```python
from build123d import *

# Parameters (mm, degrees)
SKETCH3_R            = 31
SKETCH3_R_2          = 1.6
SERVO_MOUNT_DEPTH    = 2
SKETCH4_R            = 31
SKETCH4_R_2          = 24
SPACER_DEPTH         = 9.3
FLEX_CABLE_REACH     = 47.274
SKETCH5_W            = 17
SKETCH5_H            = 0.8
SKETCH7_W            = 24
SKETCH7_H            = 62
CUT_EXTRUDE3_DEPTH   = 45.816180114
SKETCH8_W            = 62
SKETCH8_H            = 24
CUT_EXTRUDE4_DEPTH   = 45.816180114
MOUNTING_HOLES_REACH = 47.274
SKETCH10_R           = 1.4
CUT_EXTRUDE5_REACH   = 46.816
FILLET2_R            = 5


with BuildPart() as part:
    # Sketch3 → Servo mount (new body)
    with BuildSketch(Plane(origin=(0, 0, 0), x_dir=(1, 0, 0), z_dir=(0, 1, 0))):
        with Locations(Location((0, 0, 0), (0, 0, 270))):
            Circle(SKETCH3_R)
        with Locations(Location((0, -8.65, 0), (0, 0, 270))):
            Circle(SKETCH3_R_2, mode=Mode.SUBTRACT)
        with Locations(Location((0, 19.05, 0), (0, 0, 270))):
            Circle(SKETCH3_R_2, mode=Mode.SUBTRACT)
        Polygon((-6.2, 16.1), (-6.2, 2.227105745), (-6.2, -6.4), (-5.7, -6.4), (5.7, -6.4), (6.2, -6.4), (6.2, 2.227105745), (6.2, 16.1), (6.2, 16.8), (5.7, 16.8), (-5.7, 16.8), (-6.2, 16.8), align=None, mode=Mode.SUBTRACT)
    extrude(amount=-SERVO_MOUNT_DEPTH)

    # Sketch4 → Spacer (add)
    with BuildSketch(Plane(origin=(0, -2, 0), x_dir=(-1, 0, 0), z_dir=(0, -1, 0))):
        with Locations(Location((0, 0, 0), (0, 0, 270))):
            Circle(SKETCH4_R)
        with Locations(Location((0, 0, 0), (0, 0, 270))):
            Circle(SKETCH4_R_2, mode=Mode.SUBTRACT)
    extrude(amount=SPACER_DEPTH)

    # Sketch5 → Flex cable (cut, up to next)
    with BuildSketch(Plane(origin=(0, 0, 0), x_dir=(1, 0, 0), z_dir=(0, 1, 0)), mode=Mode.PRIVATE) as flex_cable_sk1:
        with Locations((0, -19.15054858)):
            Rectangle(SKETCH5_W, SKETCH5_H)
    flex_cable_tool1 = extrude(flex_cable_sk1.sketch, amount=-FLEX_CABLE_REACH, mode=Mode.PRIVATE) & part.part
    add(flex_cable_tool1.solids().sort_by_distance((0, 0, 19.150549))[0], mode=Mode.SUBTRACT)

    # Sketch7 → Cut-Extrude3 (cut, through all)
    with BuildSketch(Plane.XZ.offset(2)):
        Rectangle(SKETCH7_W, SKETCH7_H)
    extrude(amount=CUT_EXTRUDE3_DEPTH, mode=Mode.SUBTRACT)

    # Sketch8 → Cut-Extrude4 (cut, through all)
    with BuildSketch(Plane.XZ.offset(2)):
        Rectangle(SKETCH8_W, SKETCH8_H)
    extrude(amount=CUT_EXTRUDE4_DEPTH, mode=Mode.SUBTRACT)

    # Sketch10 → Mounting holes (cut, up to next)
    with BuildSketch(Plane.XZ.offset(11.3), mode=Mode.PRIVATE) as mounting_holes_sk1:
        with Locations(Location((-19.445436483, -19.445436483, 0), (0, 0, 270))):
            Circle(SKETCH10_R)
    mounting_holes_tool1 = extrude(mounting_holes_sk1.sketch, amount=-MOUNTING_HOLES_REACH, mode=Mode.PRIVATE) & part.part
    # Sketch10 → Mounting holes (cut, up to next)
    with BuildSketch(Plane.XZ.offset(11.3), mode=Mode.PRIVATE) as mounting_holes_sk2:
        with Locations(Location((19.445436483, -19.445436483, 0), (0, 0, 270))):
            Circle(SKETCH10_R)
    mounting_holes_tool2 = extrude(mounting_holes_sk2.sketch, amount=-MOUNTING_HOLES_REACH, mode=Mode.PRIVATE) & part.part
    # Sketch10 → Mounting holes (cut, up to next)
    with BuildSketch(Plane.XZ.offset(11.3), mode=Mode.PRIVATE) as mounting_holes_sk3:
        with Locations(Location((-19.445436483, 19.445436483, 0), (0, 0, 270))):
            Circle(SKETCH10_R)
    mounting_holes_tool3 = extrude(mounting_holes_sk3.sketch, amount=-MOUNTING_HOLES_REACH, mode=Mode.PRIVATE) & part.part
    # Sketch10 → Mounting holes (cut, up to next)
    with BuildSketch(Plane.XZ.offset(11.3), mode=Mode.PRIVATE) as mounting_holes_sk4:
        with Locations(Location((19.445436483, 19.445436483, 0), (0, 0, 270))):
            Circle(SKETCH10_R)
    mounting_holes_tool4 = extrude(mounting_holes_sk4.sketch, amount=-MOUNTING_HOLES_REACH, mode=Mode.PRIVATE) & part.part
    add(mounting_holes_tool1.solids().sort_by_distance((-19.445436, -11.3, -19.445436))[0], mode=Mode.SUBTRACT)
    add(mounting_holes_tool2.solids().sort_by_distance((19.445436, -11.3, -19.445436))[0], mode=Mode.SUBTRACT)
    add(mounting_holes_tool3.solids().sort_by_distance((-19.445436, -11.3, 19.445436))[0], mode=Mode.SUBTRACT)
    add(mounting_holes_tool4.solids().sort_by_distance((19.445436, -11.3, 19.445436))[0], mode=Mode.SUBTRACT)

    # Sketch11 → Cut-Extrude5 (cut, up to next)
    with BuildSketch(Plane.XZ.offset(2), mode=Mode.PRIVATE) as cut_extrude5_sk1:
        with BuildLine():
            Line((-12, -22.784609691), (12, -22.784609691))
            Line((12, -22.784609691), (12, -28.583211856))
            ThreePointArc((12, -28.583211856), (0, -31), (-12, -28.583211856))
            Line((-12, -28.583211856), (-12, -22.784609691))
        make_face()
    cut_extrude5_tool1 = extrude(cut_extrude5_sk1.sketch, amount=-CUT_EXTRUDE5_REACH, mode=Mode.PRIVATE) & part.part
    # Sketch11 → Cut-Extrude5 (cut, up to next)
    with BuildSketch(Plane.XZ.offset(2), mode=Mode.PRIVATE) as cut_extrude5_sk2:
        with BuildLine():
            Line((28.583211856, 12), (20.784609691, 12))
            Line((20.784609691, 12), (20.784609691, -12))
            Line((20.784609691, -12), (28.583211856, -12))
            ThreePointArc((28.583211856, -12), (31, 0), (28.583211856, 12))
        make_face()
    cut_extrude5_tool2 = extrude(cut_extrude5_sk2.sketch, amount=-CUT_EXTRUDE5_REACH, mode=Mode.PRIVATE) & part.part
    # Sketch11 → Cut-Extrude5 (cut, up to next)
    with BuildSketch(Plane.XZ.offset(2), mode=Mode.PRIVATE) as cut_extrude5_sk3:
        with BuildLine():
            Line((-28.583211856, -12), (-20.784609691, -12))
            Line((-20.784609691, -12), (-20.784609691, 12))
            Line((-20.784609691, 12), (-28.583211856, 12))
            ThreePointArc((-28.583211856, 12), (-31, 0), (-28.583211856, -12))
        make_face()
    cut_extrude5_tool3 = extrude(cut_extrude5_sk3.sketch, amount=-CUT_EXTRUDE5_REACH, mode=Mode.PRIVATE) & part.part
    # Sketch11 → Cut-Extrude5 (cut, up to next)
    with BuildSketch(Plane.XZ.offset(2), mode=Mode.PRIVATE) as cut_extrude5_sk4:
        with BuildLine():
            Line((12, 20.784609691), (12, 28.583211856))
            ThreePointArc((12, 28.583211856), (0, 31), (-12, 28.583211856))
            Line((-12, 28.583211856), (-12, 20.784609691))
            Line((-12, 20.784609691), (12, 20.784609691))
        make_face()
    cut_extrude5_tool4 = extrude(cut_extrude5_sk4.sketch, amount=-CUT_EXTRUDE5_REACH, mode=Mode.PRIVATE) & part.part
    add(cut_extrude5_tool1.solids().sort_by_distance((0, -2, -26.530561))[0], mode=Mode.SUBTRACT)
    add(cut_extrude5_tool2.solids().sort_by_distance((25.523226, -2, 0))[0], mode=Mode.SUBTRACT)
    add(cut_extrude5_tool3.solids().sort_by_distance((-25.523226, -2, 0))[0], mode=Mode.SUBTRACT)
    add(cut_extrude5_tool4.solids().sort_by_distance((0, -2, 25.523226))[0], mode=Mode.SUBTRACT)

    # Fillet2
    # the kernel refuses this fillet: 5 mm, written as the material it takes off along each edge
    with BuildSketch(Plane(origin=(12, -35.215595033, 28.583211856), x_dir=(0.8512708603213988, -2.9625112876132807e-14, -0.5247265215020731), z_dir=(0, 1, 0))) as fillet2_piece_1:
        with BuildLine():
            CenterArc((8.794767206, 4.940124775), FILLET2_R, 160.140208495, 118.735653745)
            Line((4.092133387, 6.638722774), (0, 0))
            ThreePointArc((0, 0), (4.783119007, -0.371226395), (9.566238013, 0))
        make_face()
    extrude(amount=59.131190067, mode=Mode.SUBTRACT)
    with BuildSketch(Plane(origin=(12, 23.915595033, -28.583211856), x_dir=(0, 0, 1), z_dir=(0, -1, 0))) as fillet2_piece_2_section:
        with BuildLine():
            CenterArc((8.820231871, -4.894514557), FILLET2_R, 101.790043136, 118.735653745)
            ThreePointArc((5.019658797, -8.143459664), (2.193815186, -4.266522167), (0, 0))
            Line((0, 0), (7.798602165, 0))
        make_face()
    fillet2_piece_2 = extrude(amount=59.131190067, mode=Mode.PRIVATE)
    fillet2_piece_2 = split(fillet2_piece_2, bisect_by=Plane(origin=(16.358047436, -1, -22.784609691), z_dir=(0, 0, -1)), keep=Keep.TOP, mode=Mode.PRIVATE)
    add(fillet2_piece_2, mode=Mode.SUBTRACT)
    with BuildSketch(Plane(origin=(12, 23.915595033, -28.583211856), x_dir=(0, 0, 1), z_dir=(0, -1, 0))) as fillet2_piece_3_section:
        with BuildLine():
            CenterArc((8.820231871, -4.894514557), FILLET2_R, 101.790043136, 118.735653745)
            ThreePointArc((5.019658797, -8.143459664), (2.193815186, -4.266522167), (0, 0))
            Line((0, 0), (7.798602165, 0))
        make_face()
    fillet2_piece_3 = extrude(amount=59.131190067, mode=Mode.PRIVATE)
    fillet2_piece_3 = split(fillet2_piece_3, bisect_by=Plane(origin=(12.335072, -2, -21.839415291), z_dir=(0, -1, 0)), keep=Keep.TOP, mode=Mode.PRIVATE)
    add(fillet2_piece_3, mode=Mode.SUBTRACT)
    with BuildSketch(Plane(origin=(28.583211856, 23.915595033, -12), x_dir=(-1, 0, 0), z_dir=(0, -1, 0))) as fillet2_piece_4:
        with BuildLine():
            CenterArc((8.820231871, 4.894514557), FILLET2_R, 139.474303119, 118.735653745)
            ThreePointArc((5.019658797, 8.143459664), (2.193815186, 4.266522167), (0, 0))
            Line((0, 0), (7.798602165, 0))
        make_face()
    extrude(amount=59.131190067, mode=Mode.SUBTRACT)
    with BuildSketch(Plane(origin=(-28.583211856, 23.915595033, -12), x_dir=(1, 0, 0), z_dir=(0, -1, 0)), Plane(origin=(28.583211856, 23.915595033, 12), x_dir=(-1, 0, 0), z_dir=(0, -1, 0))) as fillet2_piece_5:
        with BuildLine():
            CenterArc((8.820231871, -4.894514557), FILLET2_R, 101.790043136, 118.735653745)
            ThreePointArc((5.019658797, -8.143459664), (2.193815186, -4.266522167), (0, 0))
            Line((0, 0), (7.798602165, 0))
        make_face()
    extrude(amount=59.131190067, mode=Mode.SUBTRACT)
    with BuildSketch(Plane(origin=(-28.583211856, 23.915595033, 12), x_dir=(0.5247265215020732, -2.488832337515826e-14, 0.8512708603213986), z_dir=(0, -1, 0)), Plane(origin=(-12, -35.215595033, 28.583211856), x_dir=(-0.8512708603213989, -3.062415803150537e-14, -0.524726521502073), z_dir=(0, 1, 0))) as fillet2_piece_6:
        with BuildLine():
            CenterArc((8.794767206, -4.940124775), FILLET2_R, 81.12413776, 118.735653745)
            Line((4.092133387, -6.638722774), (0, 0))
            ThreePointArc((0, 0), (4.783119007, 0.371226395), (9.566238013, 0))
        make_face()
    extrude(amount=59.131190067, mode=Mode.SUBTRACT)
    with BuildSketch(Plane(origin=(-12, 23.915595033, -28.583211856), x_dir=(-0.8512708603213988, 1.214076701840839e-14, 0.5247265215020731), z_dir=(0, -1, 0))) as fillet2_piece_7_section:
        with BuildLine():
            CenterArc((8.794767206, -4.940124775), FILLET2_R, 81.12413776, 118.735653745)
            Line((4.092133387, -6.638722774), (0, 0))
            ThreePointArc((0, 0), (4.783119007, 0.371226395), (9.566238013, 0))
        make_face()
    fillet2_piece_7 = extrude(amount=59.131190067, mode=Mode.PRIVATE)
    fillet2_piece_7 = split(fillet2_piece_7, bisect_by=Plane(origin=(-16.358047436, -1, -22.784609691), z_dir=(0, 0, -1)), keep=Keep.TOP, mode=Mode.PRIVATE)
    add(fillet2_piece_7, mode=Mode.SUBTRACT)
    with BuildSketch(Plane(origin=(-12, 23.915595033, -28.583211856), x_dir=(-0.8512708603213988, 1.214076701840839e-14, 0.5247265215020731), z_dir=(0, -1, 0))) as fillet2_piece_8_section:
        with BuildLine():
            CenterArc((8.794767206, -4.940124775), FILLET2_R, 81.12413776, 118.735653745)
            Line((4.092133387, -6.638722774), (0, 0))
            ThreePointArc((0, 0), (4.783119007, 0.371226395), (9.566238013, 0))
        make_face()
    fillet2_piece_8 = extrude(amount=59.131190067, mode=Mode.PRIVATE)
    fillet2_piece_8 = split(fillet2_piece_8, bisect_by=Plane(origin=(-12.335072, -2, -21.839415291), z_dir=(0, -1, 0)), keep=Keep.TOP, mode=Mode.PRIVATE)
    add(fillet2_piece_8, mode=Mode.SUBTRACT)


solid = part.part
```
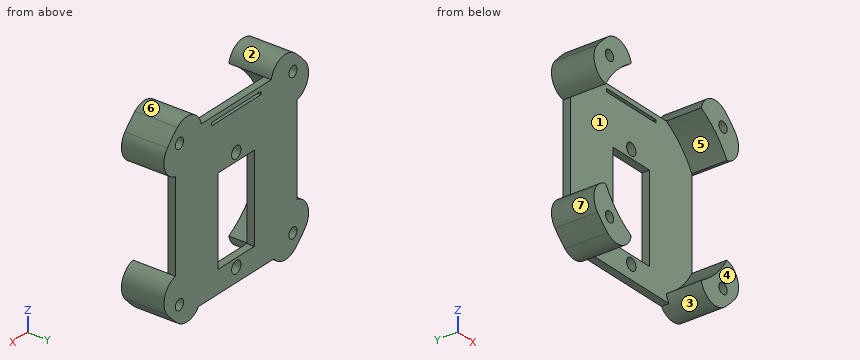
Geometry check sheet. Reference: the model listing, model coordinates, mm. Face numbers are marked on the shaded views. A direction names the side the tool comes from. Give positions to 0.01 mm unless a question says otherwise; leave off trailing zeros. Write each loop counter-clockwise with the first axis right and the second up, starting at its lowest first coordinate (ties: lowest second). Pieces come first, ordered by that corner, then holes. Notation, with made-up numbers: (-4.5, -9) - (31.5, -9) arc R33 ccw to (31.5, 26) - close; hole circle Ø6 at (8.25, -8.5). An arc over 180 degrees is marked (long way). Use a Markdown table: item, result.
Q1. Thickness scan on L1, parallel to Z at x = -2.5, y = -0.75; L2, parallel to Z at x = 19.5, y = -1.5; L3, parallel to Z at x = 20.5, y = -8.25. Record the ranges inside material, lowest first. Write a range as [from, to].
Computed:
| item | result |
|---|---|
| L1 | z = [-22.78, -16.8], [6.4, 18.75], [19.55, 20.78] |
| L2 | z = [-24.03, -20.84], [-18.05, 18.05], [20.84, 24.03] |
| L3 | z = [-23.25, -20.37], [-18.52, -12.48], [12.48, 18.52], [20.37, 23.25] |
Q2. Section check B-B, the plane x = 3.5. Enter the section's corners in (y, z).
Computed:
| item | result |
|---|---|
| outline | (-2, -22.78) - (0, -22.78) - (0, -16.8) - (-2, -16.8) - close; (-2, 6.4) - (0, 6.4) - (0, 18.75) - (-2, 18.75) - close; (-2, 19.55) - (0, 19.55) - (0, 20.78) - (-2, 20.78) - close |
Q3. Go/stop test with flat-tipped pins: P1, Ø1.6, axis at y = -1, z = -4.5, coming from the +X side; P2, Ø2, axis at x = -3.5, y = -1, coming from the +Z side; P3, Ø21, axis at x = 7, z = -2, coming from the -Y side. Record where each tip stops, or that it passes through.
Computed:
| item | result |
|---|---|
| P1 | stops at x = 20.78 |
| P2 | stops at z = 20.78 |
| P3 | stops at y = -2 |
Q4. Set-up check for the marked faces 1, 2 and 3: record each of +Z, -Z, +X, -X, +Y, -Y from which the full face is reachable in a straight line by a thin tool's end or side.
Computed:
| item | result |
|---|---|
| face 1 | -Y |
| face 2 | +Z, +Y, -Y |
| face 3 | -Z, -Y |
Q5. Section check D-D, the plane z = -19.05. Enter the section's corners in (x, y), then the cut area to 3 significant figures.
Computed:
| item | result |
|---|---|
| outline | (-24.27, -11.3) - (-20.79, -11.3) - (-20.79, 0) - (-24.27, 0) - close; (-18.1, -11.3) - (-14.6, -11.3) - (-14.6, -2) - (-1.6, -2) - (-1.6, 0) - (-18.1, 0) - close; (1.6, -2) - (14.6, -2) - (14.6, -11.3) - (18.1, -11.3) - (18.1, 0) - (1.6, 0) - close; (20.79, -11.3) - (24.27, -11.3) - (24.27, 0) - (20.79, 0) - close |
| area | 210 mm² |
Q6. Section check A-A, the plane z = 8.65. Enter the section's corners in (x, y).
Computed:
| item | result |
|---|---|
| outline | (-20.78, -2) - (-1.6, -2) - (-1.6, 0) - (-20.78, 0) - close; (1.6, -2) - (20.78, -2) - (20.78, 0) - (1.6, 0) - close |
Q7. Section check C-C, the plane y = -4.5. Enter the section's corners in (x, z), then the cut area to 3 significant figures.
Computed:
| item | result |
|---|---|
| outline | (-23.56, -20.14) arc R31 ccw to (-20.14, -23.56) arc R5 ccw to (-12, -20.78) arc R24 cw to (-20.78, -12) arc R5 ccw to start; (-23.56, 20.14) arc R5 ccw to (-20.78, 12) arc R24 cw to (-12, 20.78) arc R5 ccw to (-20.14, 23.56) arc R31 ccw to start; (12, -20.78) arc R5 ccw to (20.14, -23.56) arc R31 ccw to (23.56, -20.14) arc R5 ccw to (20.78, -12) arc R24 cw to start; (12, 20.78) arc R24 cw to (20.78, 12) arc R5 ccw to (23.56, 20.14) arc R31 ccw to (20.14, 23.56) arc R5 ccw to start; hole circle Ø2.8 at (-19.45, -19.45); hole circle Ø2.8 at (-19.45, 19.45); hole circle Ø2.8 at (19.45, -19.45); hole circle Ø2.8 at (19.45, 19.45) |
| area | 336 mm² |
Q8. Draft check along Z on the marked faces 4, 5, 6 and 7. Enter one of: pulls with the +Z half, pulls with the -Z half, needs draft (parallel to the pull), parting line crosses it, or undercut.
Computed:
| item | result |
|---|---|
| face 4 | needs draft |
| face 5 | undercut |
| face 6 | pulls with the +Z half |
| face 7 | undercut |
